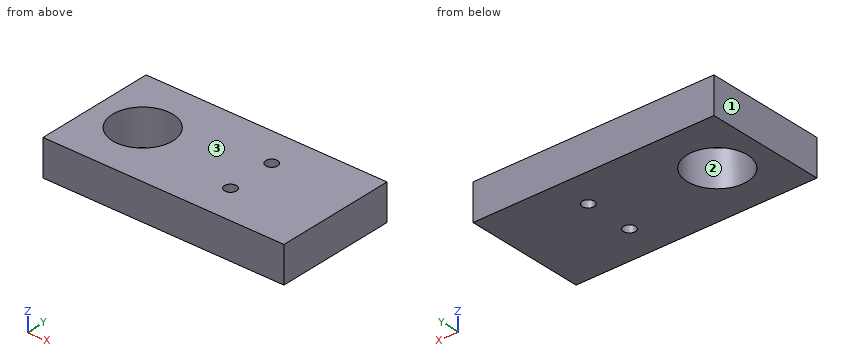
Autodesk Inventor part; units mm, degrees
ref_plane "YZ Plane" through (0, 0, 0) normal (1, 0, 0) x (0, 1, 0)
ref_plane "XZ Plane" through (0, 0, 0) normal (0, 1, 0) x (-1, 0, 0)
ref_plane "XY Plane" through (0, 0, 0) normal (0, 0, 1) x (1, 0, 0)
sketch "Sketch1" plane through (0, 0, 0) normal (0, 0, 1) x (1, 0, 0)
  line L0 (0, 0) -> (20, 0)
  line L1 (20, 0) -> (20, 10)
  line L2 (20, 10) -> (0, 10)
  line L3 (0, 10) -> (0, 0)
  circle A0 centre (4, 5) radius 2.5
  circle A1 centre (13, 3) radius 0.5
  circle A2 centre (13, 7) radius 0.5
  point P0 (0, 5)
  dimension "d0" = 20
  dimension "d1" = 10
  dimension "d3" = 5
  dimension "d4" = 4
  dimension "d7" = 1
  dimension "d8" = 1
  dimension "d9" = 4
  dimension "d10" = 3
  dimension "d11" = 13
extrude "Extrusión1" add sketch "Sketch1" along normal blind 3
Can you work these out from the model? Positions are in its coordinate system, mm. Face numbers are marked on the shaded views. Coordinates: 2 decimals unless noted, no trailing zeros. Loops run counter-clockwise (first coordinate to the right, second up) from the corner with the lowest first, then second, coordinate; pieces in that order, holes last. Notation, with made-up numbers: (30, -27.5) - (43, -27.5) arc R18 cw to (43, -14.5) - close; hole circle Ø6 at (-33.75, 19.5). An arc over 180 degrees is marked (long way). Put each result on its own line as item: value. Start each with the question number.
Item 1: Suppose I cut it at A-A (y = 5). Please give me the cut outline in (x, z).
Item 2: Suppose I cut it at B-B (x = 2.5). Please give me the cut outline in (y, z), and give its area (3 significant figures).
Item 3: If I drill on line 1 along Y through (x, z) = (13, 1.7); line 2 along Y through (x, z) = (6, 0.2); line 3 along Y through (x, z) = (4, 1.8), over which ranges is the centre line in solid material (lowest first)?
Item 4: If we mould it in two halves opening along X, with no side actions, what happens to the marked faces 1, 2 and 3? For each: +X half, -X half, draft (parallel to the pull), parting line (faces both ways), or undercut.
Item 5: Suppose I cut it at D-D (y = 3). Please give me the cut outline in (x, z), and give its area (3 significant figures).
Item 6: Suppose I cut it at C-C (z = 2.8). Please give me the cut outline in (x, y).
Here are the results:
1. outline: (0, 0) - (1.5, 0) - (1.5, 3) - (0, 3) - close; (6.5, 0) - (20, 0) - (20, 3) - (6.5, 3) - close
2. outline: (0, 0) - (3, 0) - (3, 3) - (0, 3) - close; (7, 0) - (10, 0) - (10, 3) - (7, 3) - close
2. area: 18.0 mm²
3. line 1: 0 to 2.5, 3.5 to 6.5, 7.5 to 10
3. line 2: 0 to 3.5, 6.5 to 10
3. line 3: 0 to 2.5, 7.5 to 10
4. face 1: -X half
4. face 2: undercut
4. face 3: draft
5. outline: (0, 0) - (2.5, 0) - (2.5, 3) - (0, 3) - close; (5.5, 0) - (12.5, 0) - (12.5, 3) - (5.5, 3) - close; (13.5, 0) - (20, 0) - (20, 3) - (13.5, 3) - close
5. area: 48.0 mm²
6. outline: (0, 0) - (20, 0) - (20, 10) - (0, 10) - close; hole circle Ø5 at (4, 5); hole circle Ø1 at (13, 3); hole circle Ø1 at (13, 7)
